from build123d import *

# Parameters (mm, degrees)
F0_R     = 2.5
F0_R_2   = 2
F0_W     = 21.32
F0_H     = 41.64
F1_DEPTH = 5


with BuildPart() as f1:
    # F0 (on Top) → F1 (new body)
    with BuildSketch(Plane.XY):
        with BuildLine():
            Line((30, 50), (-30, 50))
            ThreePointArc((-30, 50), (-33.535534, 48.535534), (-35, 45))
            Line((-35, 45), (-35, -45))
            ThreePointArc((-35, -45), (-33.535534, -48.535534), (-30, -50))
            Line((-30, -50), (30, -50))
            ThreePointArc((30, -50), (33.535534, -48.535534), (35, -45))
            Line((35, -45), (35, 45))
            ThreePointArc((35, 45), (33.535534, 48.535534), (30, 50))
        make_face()
        with Locations((-25, -40)):
            Circle(F0_R, mode=Mode.SUBTRACT)
        with Locations((-5.085, -34.29)):
            Circle(F0_R_2, mode=Mode.SUBTRACT)
        with Locations((5.085, -34.29)):
            Circle(F0_R_2, mode=Mode.SUBTRACT)
        with Locations((25, -40)):
            Circle(F0_R, mode=Mode.SUBTRACT)
        with Locations((0, -10.16)):
            Rectangle(F0_W, F0_H, mode=Mode.SUBTRACT)
        with Locations((-5.085, 13.97)):
            Circle(F0_R_2, mode=Mode.SUBTRACT)
        with Locations((-25, 40)):
            Circle(F0_R, mode=Mode.SUBTRACT)
        with Locations((5.085, 13.97)):
            Circle(F0_R_2, mode=Mode.SUBTRACT)
        with Locations((25, 40)):
            Circle(F0_R, mode=Mode.SUBTRACT)
    extrude(amount=F1_DEPTH)


solid = f1.part
Read the model definition and answer for the solid it produces. Units are mm, in the model's axes. A direction names the side the tool comes from. Round coordinates to 2 decimals unless told otherwise and drop trailing zeros. Loops run counter-clockwise (first coordinate to the right, second up) from the corner with the lowest first, then second, coordinate; pieces in that order, holes last.
Q1. Consider probe 1 along Y at (x, z) = (25, 3.9); probe 2 along Y at (x, z) = (2, 4.25); probe 3 along Y at (x, z) = (6, 3.8). Determine where each line is inside the solid, lowest interval first.
Q2. Which of the six approach directions +Z, -Z, +X, -X, +Y, -Y give full straight-line access (tool end or side, diameter ignored) to faces 1 (the face through (0, -30.98, 2)), 2 (the face through (0, 50, 2))?
Q3. Determine the mould class of faces 3 (the face through (10.66, -10, 2)), 4 (the face through (0, -50, 2)), 5 (the face through (-5.345, 15.953, 2.465)), 6 (the face through (34, 48, 2)) for opening direction X: released by +X, released by -X, zero draft, split by the parting line, or undercut.
Q4. Section A-A on x = -9.5 is taken. Write down the section's boundary in (y, z), and give its area (3 significant figures).
Q5. Section D-D on z = 4.15 is taken. Give the number of separate pieces and of enclosed holes in the cut face, and give its area (3 significant figures).
Q6. Section B-B on y = 13.97 is taken. Write down the section's boundary in (x, z) (3 decimals), and give its area (3 significant figures).
Q7. Each of these flat-tipped pins is pushed along its axis until it touches: pin 1 (6.5 mm diameter, centred on x = -25, y = -40, fed in from +Z); pin 2 (3 mm diameter, centred on x = 5.085, y = 13.97, fed in from +Z) (1 decimal). Where does it stop, or does it pass through?
Q8. Section C-C on x = 25 is taken. Write down the section's boundary in (y, z), and give its area (3 significant figures).
Output:
1. probe 1: y = -50 to -42.5, -37.5 to 37.5, 42.5 to 50
1. probe 2: y = -50 to -30.98, 10.66 to 50
1. probe 3: y = -50 to -36.07, -32.51 to -30.98, 10.66 to 12.19, 15.75 to 50
2. face 1: +Z, -Z
2. face 2: +Z, -Z, +X, -X, +Y
3. face 3: undercut
3. face 4: zero draft
3. face 5: undercut
3. face 6: released by +X
4. outline: (-50, 0) - (-30.98, 0) - (-30.98, 5) - (-50, 5) - close; (10.66, 0) - (50, 0) - (50, 5) - (10.66, 5) - close
4. area: 292 mm2
5. separate pieces: 1
5. enclosed holes: 9
5. area: 5,960 mm2
6. outline: (-35, 0) - (-7.085, 0) - (-7.085, 5) - (-35, 5) - close; (-3.085, 0) - (3.085, 0) - (3.085, 5) - (-3.085, 5) - close; (7.085, 0) - (35, 0) - (35, 5) - (7.085, 5) - close
6. area: 310 mm2
7. pin 1: stops at z = 5
7. pin 2: passes through
8. outline: (-50, 0) - (-42.5, 0) - (-42.5, 5) - (-50, 5) - close; (-37.5, 0) - (37.5, 0) - (37.5, 5) - (-37.5, 5) - close; (42.5, 0) - (50, 0) - (50, 5) - (42.5, 5) - close
8. area: 450 mm2
